The listing builds one solid part. Answer for the finished solid, in the listing's coordinates (mm). A direction names the side the tool comes from. Coordinates: 2 decimals unless noted, no trailing zeros. Loops run counter-clockwise (first coordinate to the right, second up) from the corner with the lowest first, then second, coordinate; pieces in that order, holes last. Notation, with made-up numbers: M 24,-12.75 L 33,-12.75 A21 ccw 33,11.25 Z; hole C 86,-6.5 d8. An arc over 180 degrees is marked long. Return JSON: item names as keys, results as strings. Group by question number.
1. Section B-B (y = 2.25) is taken. Write down the section's boundary in (x, z), then the cut area to 3 significant figures.
2. Given P1, Ø1.5, axis at y = 1.5, z = 9.5, coming from the -X side; P2, Ø1.5, axis at x = -2, y = 1.5, coming from the -Z side; P3, Ø1, axis at x = 27.5, y = 0.5, coming from the -Z side; P4, Ø2, axis at x = 27.5, z = -18, coming from the -Y side, each flat-ended and moving along its own axis, determine where each tip first touches the part or whether it passes through.
3. Straight lines are drawn through the part: L1, parallel to X at y = 2.5, z = -15; L2, parallel to Z at x = -24, y = 0.7; L3, parallel to Z at x = -24, y = 1.75. For each, find the intervals that lie inside material, in ascending order. Write a range as from..to.
4. Section A-A (z = 0) is taken. Write down the section's boundary in (x, y), then the cut area to 3 significant figures.
5. Which of the six approach directions +Z, -Z, +X, -X, +Y, -Y give full straight-line access (tool end or side, diameter ignored) to faces 1 (the face through (1.517, 2.24, -34.467)), 2 (the face through (0, 3, 0))?
```python
from build123d import *

# Parameters (mm, degrees)
SKETCH1_R           = 37.5
BOSS_EXTRUDE1_DEPTH = 1
SKETCH2_R           = 34.5
BOSS_EXTRUDE2_DEPTH = 3
FILLET1_R           = 5
SKETCH3_R           = 37.5
BOSS_EXTRUDE3_DEPTH = 0.5


with BuildPart() as part:
    # Sketch1 → Boss-Extrude1 (new body)
    with BuildSketch(Plane(origin=(0, 0, 0), x_dir=(1, 0, 0), z_dir=(0, 1, 0))):
        with Locations(Location((0, 0, 0), (0, 0, 270))):
            Circle(SKETCH1_R)
    extrude(amount=BOSS_EXTRUDE1_DEPTH)

    # Sketch2 → Boss-Extrude2 (add)
    with BuildSketch(Plane(origin=(0, 0, 0), x_dir=(1, 0, 0), z_dir=(0, 1, 0))):
        with Locations(Location((0, 0, 0), (0, 0, 270))):
            Circle(SKETCH2_R)
    extrude(amount=BOSS_EXTRUDE2_DEPTH)

    # Fillet1
    # the kernel refuses this fillet: 5 mm, written as the material it takes off along each edge
    with BuildSketch(Plane(origin=(0, 0, 0), x_dir=(0, 0, 1), z_dir=(-1, 0, 0))) as fillet1_piece_1:
        with BuildLine():
            CenterArc((34.5, 5), FILLET1_R, 270, 36.869897646)
            Line((34.5, 0), (34.5, -0.1))
            Line((34.5, -0.1), (37.5, -0.1))
            Line((37.5, -0.1), (37.6, 0))
            ThreePointArc((37.6, 0), (37.6, 0.5), (37.56, 0.92))
            Line((37.56, 0.92), (37.5, 1))
        make_face()
    revolve(axis=Axis((0, 0, 0), (0, 1, 0)), mode=Mode.SUBTRACT)

    # Sketch3 → Boss-Extrude3 (add)
    with BuildSketch(Plane(origin=(0, 1, 0), x_dir=(1, 0, 0), z_dir=(0, 1, 0))):
        with Locations(Location((0, 0, 0), (0, 0, 270))):
            Circle(SKETCH3_R)
    extrude(amount=BOSS_EXTRUDE3_DEPTH)


solid = part.part
```
Worked out:
{
 "1": {"outline": "C 0,0 d69", "area": "3,740 mm^2"},
 "2": {"P1": "x = -36.46", "P2": "z = -37.48", "P3": "z = -25.63", "P4": "y = 0"},
 "3": {"L1": "-31.07..31.07", "L2": "-28.23..28.23", "L3": "-24.78..24.78"},
 "4": {"outline": "M -37.5,1 A5 ccw -34.5,0 L 34.5,0 A5 ccw 37.5,1 L 37.5,1.5 L 34.5,1.5 L 34.5,3 L -34.5,3 L -34.5,1.5 L -37.5,1.5 Z", "area": "214 mm^2"},
 "5": {"face 1": "+Y", "face 2": "+Z, -Z, +X, -X, +Y"}
}
